Geometry: final body of the model. Coordinates: model frame, mm. Face numbers are marked on the shaded views. A direction names the side the tool comes from. Give positions to 0.01 mm unless a question says otherwise; leave off trailing zeros. Write each loop counter-clockwise with the first axis right and the second up, starting at its lowest first coordinate (ties: lowest second). Pieces come first, ordered by that corner, then holes.
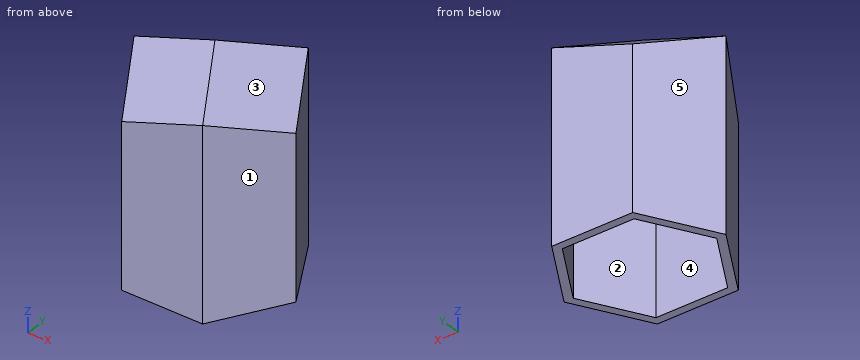
from build123d import *

# Parameters (mm, degrees)
F1_DEPTH  = 38.1
F8_W      = 62.1289778501
F8_H      = 70.9990356117
F9_DEPTH  = 24.4074275016
F10_W     = 94.4273807108
F10_H     = 95.7268364727
F11_DEPTH = 24.4074275016
F12_W     = 81.8659365177
F12_H     = 67.1387314796
F13_DEPTH = 20.7508335567
F14_T     = -2.5


with BuildPart() as f1:
    # F0 (on Top) → F1 (new body, symmetric)
    with BuildSketch(Plane.XY):
        Polygon((12.7, 21.9970452561), (-12.7, 21.9970452561), (-25.4, 0), (-12.7, -21.9970452561), (12.7, -21.9970452561), (25.4, 0), align=None)
    extrude(amount=F1_DEPTH, both=True)

    # F8 (on 3pt) → F9 (cut, through all)
    with BuildSketch(Plane(origin=(-7.2159394472, 12.5101757995, 20.4417548078), x_dir=(0.9575384102, 0.1504945841, 0.2459096848), z_dir=(0.2883057283, -0.4998317088, -0.8167301084))):
        with Locations((4.8328703269, 13.4997954592)):
            Rectangle(F8_W, F8_H)
    extrude(amount=-F9_DEPTH, mode=Mode.SUBTRACT)

    # F10 (on 3pt) → F11 (cut, through all)
    with BuildSketch(Plane(origin=(-7.2159394472, -12.5101757995, 20.4417548078), x_dir=(0.9575384102, -0.1504945841, 0.2459096848), z_dir=(0.2883057283, 0.4998317088, -0.8167301084))):
        with Locations((0.9678620845, 0.6989594549)):
            Rectangle(F10_W, F10_H)
    extrude(amount=-F11_DEPTH, mode=Mode.SUBTRACT)

    # F12 (on 3pt) → F13 (cut, through all)
    with BuildSketch(Plane(origin=(14.4326980932, 0, 20.4429151462), x_dir=(0.816922581, 0, -0.5767473422), z_dir=(-0.5767473422, 0, -0.816922581))):
        with Locations((5.5516734719, -0.7580146194)):
            Rectangle(F12_W, F12_H)
    extrude(amount=-F13_DEPTH, mode=Mode.SUBTRACT)

    # F14
    f14_openings = [f1.faces().sort_by_distance(p)[0] for p in [
        (0, 0, -38.1),
    ]]
    offset(amount=F14_T, openings=f14_openings, kind=Kind.INTERSECTION)


solid = f1.part
Q1. Section C-C on y = 11. Output: boundary loops of the cut face in (x, z), plus the area to 3 significant figures.
Filled sheet:
outline: (-19.05, -38.1) - (-16.16, -38.1) - (-16.16, 15.15) - (6.35, 23.09) - (16.16, 16.16) - (16.16, -38.1) - (19.05, -38.1) - (19.05, 17.18) - (6.34, 26.15) - (-19.05, 17.19) - close
area: 423 mm2
Q2. Pull-direction query (X, two-part tool) for the marked faces 3, 4 and 5; classes: released by +X, released by -X, zero draft, split by the parting line, or undercut.
Filled sheet:
face 3: released by +X
face 4: undercut
face 5: released by -X
Q3. Pin query (flat end, axial travel): P1, Ø1.5, axis at x = 13.5, y = 0, coming from the +Z side; P2, Ø6, axis at y = 4.5, z = 9, coming from the -X side; P3, Ø1, axis at y = -14.5, z = -21, coming from the -X side. Return the tip coordinate at first contact, or that it passes through.
Filled sheet:
P1: stops at z = 21.63
P2: stops at x = -24.53
P3: stops at x = -17.32
Q4. Section D-D on z = 14.5. Output: boundary loops of the cut face in (x, y), plus the area to 3 significant figures.
Filled sheet:
outline: (-25.4, 0) - (-15.25, -17.59) - (-7.6, -22) - (12.7, -22) - (22.85, -4.42) - (22.85, 4.42) - (12.7, 22) - (-7.6, 22) - (-15.25, 17.59) - close; hole (-22.51, 0) - (-15.25, -12.58) - (-3.26, -19.5) - (11.26, -19.5) - (18.52, -6.92) - (18.52, 6.92) - (11.26, 19.5) - (-3.26, 19.5) - (-15.25, 12.58) - close
area: 409 mm2
Q5. Access query for the marked faces 1 and 2. Directions: +Z, -Z, +X, -X, +Y, -Y. A direction counts if a zero-diameter tool reaches every point of the face in a straight line with its end or side. Return the directions, or none.
Filled sheet:
face 1: +Z, -Z, +X, -Y
face 2: -Z
Q6. Section B-B on x = 6. Output: boundary loops of the cut face in (y, z).
Filled sheet:
outline: (-22, -38.1) - (-19.5, -38.1) - (-19.5, 17.77) - (-10.4, 23.34) - (10.4, 23.34) - (19.5, 17.77) - (19.5, -38.1) - (22, -38.1) - (22, 19.3) - (10.4, 26.4) - (-10.4, 26.4) - (-22, 19.3) - close
Q7. Section A-A on z = 4. Output: boundary loops of the cut face in (x, y), plus the area to 3 significant figures.
Filled sheet:
outline: (-25.4, 0) - (-12.7, -22) - (12.7, -22) - (25.4, 0) - (12.7, 22) - (-12.7, 22) - close; hole (-22.51, 0) - (-11.26, -19.5) - (11.26, -19.5) - (22.51, 0) - (11.26, 19.5) - (-11.26, 19.5) - close
area: 359 mm2
Q8. Ray query, line 1 along Y through (x, z) = (3, -16); line 2 along Y through (x, z) = (-16, 0); line 3 along X through (y, z) = (16.5, 5.5). Return the intervals inside material, ascending.
Filled sheet:
line 1: y = -22 to -19.5, 19.5 to 22
line 2: y = -16.28 to -11.28, 11.28 to 16.28
line 3: x = -15.87 to -12.99, 12.99 to 15.87
